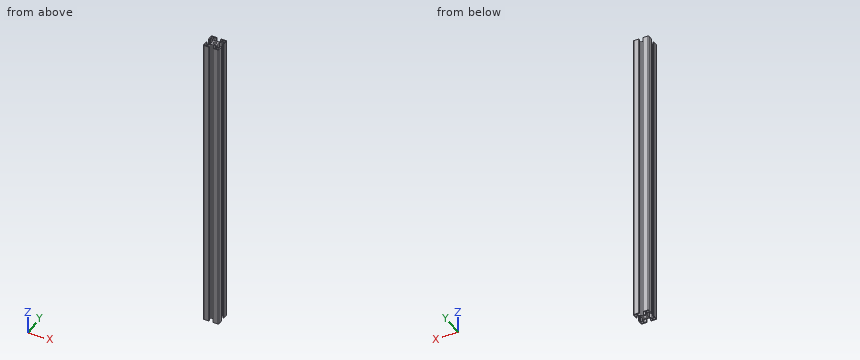
```python
from build123d import *

# Parameters (mm, degrees)
SKETCH1_R           = 2.1
SKETCH1_R_2         = 3.4
BOSS_EXTRUDE1_DEPTH = 600


with BuildPart() as part:
    # Sketch1 → Boss-Extrude1 (new body)
    with BuildSketch(Plane.XY):
        with BuildLine():
            Line((-15, -4.3), (-15, -13))
            ThreePointArc((-15, -13), (-14.414213562, -14.414213562), (-13, -15))
            Line((-13, -15), (-4.3, -15))
            ThreePointArc((-4.3, -15), (-4.087867966, -14.912132034), (-4, -14.7))
            Line((-4, -14.7), (-4, -13))
            Line((-4, -13), (-8.249996, -13))
            Line((-8.249996, -13), (-8.249996, -9.664209562))
            Line((-8.249996, -9.664209562), (-4.585786438, -6))
            Line((-4.585786438, -6), (-0.519615242, -6))
            Line((-0.519615242, -6), (0, -5.7))
            Line((0, -5.7), (0.519615242, -6))
            Line((0.519615242, -6), (4.585786438, -6))
            Line((4.585786438, -6), (8.250004, -9.664217562))
            Line((8.250004, -9.664217562), (8.250004, -13))
            Line((8.250004, -13), (4, -13))
            Line((4, -13), (4, -14.7))
            ThreePointArc((4, -14.7), (4.087867966, -14.912132034), (4.3, -15))
            Line((4.3, -15), (13, -15))
            ThreePointArc((13, -15), (14.414213562, -14.414213562), (15, -13))
            Line((15, -13), (15, -4.3))
            ThreePointArc((15, -4.3), (14.912132034, -4.087867966), (14.7, -4))
            Line((14.7, -4), (13, -4))
            Line((13, -4), (13, -8.25))
            Line((13, -8.25), (9.664213562, -8.25))
            Line((9.664213562, -8.25), (6, -4.585786438))
            Line((6, -4.585786438), (6, -0.519615242))
            Line((6, -0.519615242), (5.7, 0))
            Line((5.7, 0), (6, 0.519615242))
            Line((6, 0.519615242), (6, 4.585786438))
            Line((6, 4.585786438), (9.664213562, 8.25))
            Line((9.664213562, 8.25), (13, 8.25))
            Line((13, 8.25), (13, 4))
            Line((13, 4), (14.7, 4))
            ThreePointArc((14.7, 4), (14.912132034, 4.087867966), (15, 4.3))
            Line((15, 4.3), (15, 13))
            ThreePointArc((15, 13), (14.414213562, 14.414213562), (13, 15))
            Line((13, 15), (4.3, 15))
            ThreePointArc((4.3, 15), (4.087867966, 14.912132034), (4, 14.7))
            Line((4, 14.7), (4, 13))
            Line((4, 13), (8.25, 13))
            Line((8.25, 13), (8.25, 9.664213562))
            Line((8.25, 9.664213562), (4.585786438, 6))
            Line((4.585786438, 6), (0.519615242, 6))
            Line((0.519615242, 6), (0, 5.7))
            Line((0, 5.7), (-0.519615242, 6))
            Line((-0.519615242, 6), (-4.585786438, 6))
            Line((-4.585786438, 6), (-8.25, 9.664213562))
            Line((-8.25, 9.664213562), (-8.25, 13))
            Line((-8.25, 13), (-4, 13))
            Line((-4, 13), (-4, 14.7))
            ThreePointArc((-4, 14.7), (-4.087867966, 14.912132034), (-4.3, 15))
            Line((-4.3, 15), (-13, 15))
            ThreePointArc((-13, 15), (-14.414213562, 14.414213562), (-15, 13))
            Line((-15, 13), (-15, 4.3))
            ThreePointArc((-15, 4.3), (-14.912132034, 4.087867966), (-14.7, 4))
            Line((-14.7, 4), (-13, 4))
            Line((-13, 4), (-13, 8.25))
            Line((-13, 8.25), (-9.664213562, 8.25))
            Line((-9.664213562, 8.25), (-6, 4.585786438))
            Line((-6, 4.585786438), (-6, 0.519615242))
            Line((-6, 0.519615242), (-5.7, 0))
            Line((-5.7, 0), (-6, -0.519615242))
            Line((-6, -0.519615242), (-6, -4.585786438))
            Line((-6, -4.585786438), (-9.664213562, -8.25))
            Line((-9.664213562, -8.25), (-13, -8.25))
            Line((-13, -8.25), (-13, -4))
            Line((-13, -4), (-14.7, -4))
            ThreePointArc((-14.7, -4), (-14.912132034, -4.087867966), (-15, -4.3))
        make_face()
        with Locations((11.625, -11.625)):
            Circle(SKETCH1_R, mode=Mode.SUBTRACT)
        with Locations((11.625, 11.625)):
            Circle(SKETCH1_R, mode=Mode.SUBTRACT)
        Circle(SKETCH1_R_2, mode=Mode.SUBTRACT)
        with Locations((-11.625, -11.625)):
            Circle(SKETCH1_R, mode=Mode.SUBTRACT)
        with Locations((-11.625, 11.625)):
            Circle(SKETCH1_R, mode=Mode.SUBTRACT)
    extrude(amount=-BOSS_EXTRUDE1_DEPTH)


solid = part.part
```
The model under review builds one solid part; all positions refer to its coordinate system, in mm. Round coordinates to 2 decimals unless told otherwise and drop trailing zeros.
(1) We need section A-A on z = -491.5. Give the number of separate pieces and of enclosed holes in the cut face, and give its area (3 significant figures).
(2) Wall thickness on L1, parallel to X at y = 11, z = -165; L2, parallel to X at y = 12, z = -161.5; L3, parallel to Y at x = -4.25, z = -204: over which ranges is each line inside the solid? List them lowest first.
(3) Insertion check: pin 1 (0.8 mm diameter, centred on y = -14, z = -245, fed in from -X); pin 2 (8 mm diameter, centred on x = -4.5, y = -7, fed in from +Z); pin 3 (1.5 mm diameter, centred on x = -1, z = -77.5, fed in from -Y); pin 4 (0.8 mm diameter, centred on y = -13.5, z = -394, fed in from +X). Each pin has a flat end and moves straight along its axis. Give the tip position at first contact, or say it passes through.
Findings below:
1. separate pieces: 1
1. enclosed holes: 5
1. area: 332 mm2
2. L1: x = -15 to -13.63, -9.62 to -8.25, 8.25 to 9.62, 13.63 to 15
2. L2: x = -15 to -13.69, -9.56 to -8.25, 8.25 to 9.56, 13.69 to 15
2. L3: y = -15 to -13, -6 to 6, 13 to 15
3. pin 1: stops at x = -14.91
3. pin 2: stops at z = 0
3. pin 3: stops at y = -6
3. pin 4: stops at x = 15
